The figure shows three views and two pictorial views of one solid part (mm, origin at its lowest corner). Answer the questions. A direction names the side the tool comes from. Coordinates: 2 decimals unless noted, no trailing zeros. Order: outer loops, then holes, each group sorted by start corner. A loop starts at its lowest first (then second) coordinate and runs counter-clockwise, first axis right, second up. Notation, with made-up numbers: (67.25, 76.5) -> (123.25, 76.5) arc R18 cw to (123.25, 89.5) -> close; hole circle Ø11 at (-36, 80.25). An arc over 180 degrees is marked (long way). Return JSON: item names as keys, results as strings.
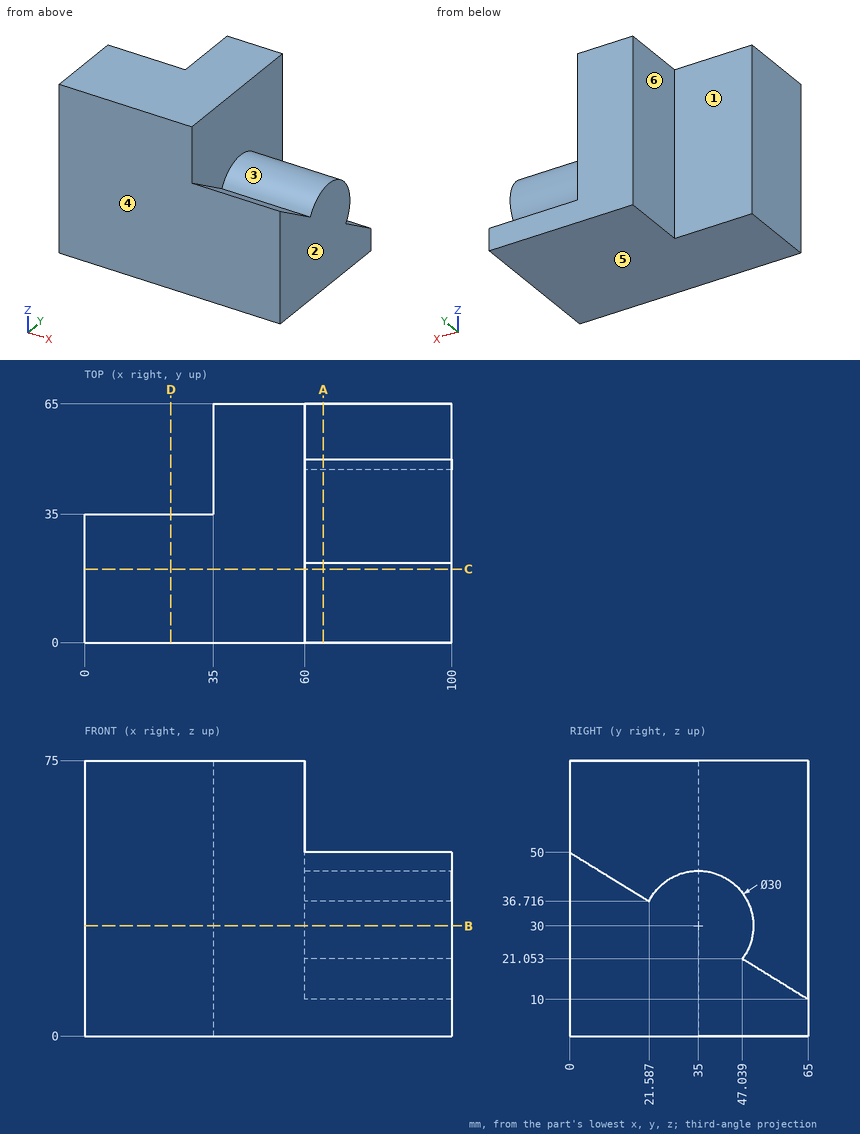
Item 1: Determine the mould class of the marked faces 1, 2, 3 and 4 for opening direction Y: pulls with the +Y half, pulls with the -Y half, needs draft (parallel to the pull), parting line crosses it, or undercut.
Answer list:
{"face 1": "pulls with the +Y half", "face 2": "needs draft", "face 3": "undercut", "face 4": "pulls with the -Y half"}
Item 2: Flat-ended cylindrical pins translate along their axes: pin 1 (19.5 mm diameter, centred on y = 43, z = 58, fed in from +X); pin 2 (17.5 mm diameter, centred on x = 19.5, z = 31, fed in from +Y); pin 3 (10 mm diameter, centred on x = 23, y = 23.5, fed in from -Z); pin 4 (24 mm diameter, centred on y = 49, z = 45, fed in from -X). Find the tip coordinate at first contact, or state that the pin passes through.
Answer list:
{"pin 1": "x = 60", "pin 2": "y = 35", "pin 3": "z = 0", "pin 4": "x = 35"}
Item 3: The part is cut by section C-C on y = 20. Determine the outline of the cut face in (x, z), plus the area to 3 significant figures.
Answer list:
{"outline": "(0, 0) -> (100, 0) -> (100, 37.69) -> (60, 37.69) -> (60, 75) -> (0, 75) -> close", "area": "6,010 mm2"}
Item 4: Which of the six approach directions +Z, -Z, +X, -X, +Y, -Y give full straight-line access (tool end or side, diameter ignored) to the marked faces 5 and 6?
Answer list:
{"face 5": "-Z, +X, -X, +Y, -Y", "face 6": "+Z, -Z, -X, +Y"}
Item 5: The part is cut by section A-A on x = 65. Determine the outline of the cut face in (y, z) (1 decimal), plus the area to 3 significant figures.
Answer list:
{"outline": "(0, 0) -> (65, 0) -> (65, 10) -> (47, 21.1) arc R15 ccw (long way) to (21.6, 36.7) -> (0, 50) -> close", "area": "2,340 mm2"}
Item 6: Find the intervals of material crossed by probe 1 along X at (y, z) = (42, 21.5); probe 2 along X at (y, z) = (54.5, 40.5); probe 3 along Y at (x, z) = (27.5, 46.5), in increasing order.
Answer list:
{"probe 1": "35 to 100", "probe 2": "35 to 60", "probe 3": "0 to 35"}
Item 7: The part is cut by section B-B on z = 30. Determine the outline of the cut face in (x, y).
Answer list:
{"outline": "(0, 0) -> (100, 0) -> (100, 50) -> (60, 50) -> (60, 65) -> (35, 65) -> (35, 35) -> (0, 35) -> close"}
Item 8: The part is cut by section D-D on x = 23.5. Determine the outline of the cut face in (y, z).
Answer list:
{"outline": "(0, 0) -> (35, 0) -> (35, 75) -> (0, 75) -> close"}
